```python
from build123d import *

# Parameters (mm, degrees)
SKETCH_1_W               = 10
SKETCH_1_H               = 10
SKETCH_1_W_2             = 8
SKETCH_1_H_2             = 8
EXTRUDE_1_DEPTH          = 121
SKETCH_2_R               = 1.5
CUT_EXTRUDE_1_DEPTH      = 11
SKETCH_3_R               = 1.5
CUT_EXTRUDE_2_DEPTH      = 51.396370289
CUT_EXTRUDE_2_DEPTH_BACK = 11.103629711


with BuildPart() as part:
    # 草图1 → 拉伸-薄壁1 (new body)
    with BuildSketch(Plane.XY):
        Rectangle(SKETCH_1_W, SKETCH_1_H)
        Rectangle(SKETCH_1_W_2, SKETCH_1_H_2, mode=Mode.SUBTRACT)
    extrude(amount=EXTRUDE_1_DEPTH)

    # 草图2 → 切除-拉伸1 (cut, through all)
    with BuildSketch(Plane(origin=(5, 0, 0), x_dir=(0, 0, -1), z_dir=(1, 0, 0))):
        with Locations((-103, 0)):
            Circle(SKETCH_2_R)
        with Locations((-35.5, 0)):
            Circle(SKETCH_2_R)
        with Locations((-25.5, 0)):
            Circle(SKETCH_2_R)
        with Locations((-93, 0)):
            Circle(SKETCH_2_R)
        Polygon((-112.339745962, 0), (-103.679491924, 5), (-121, 5), (-121, -5), (-109.452994616, -5), align=None)
        Polygon((-8.660254038, 0), (-17.320508076, -5), (0, -5), (0, 5), (-11.547005384, 5), align=None)
    extrude(amount=-CUT_EXTRUDE_1_DEPTH, mode=Mode.SUBTRACT)

    # 草图3 → 切除-拉伸2 (cut, two sides)
    with BuildSketch(Plane(origin=(0, 8.75, 5.051814855), x_dir=(1, 0, 0), z_dir=(0, 0.866025404, 0.5))) as cut_extrude_2_sk:
        with Locations((0, -12)):
            Circle(SKETCH_3_R)
    extrude(amount=CUT_EXTRUDE_2_DEPTH, mode=Mode.SUBTRACT)
    extrude(cut_extrude_2_sk.sketch, amount=-CUT_EXTRUDE_2_DEPTH_BACK, mode=Mode.SUBTRACT)


solid = part.part
```
Can you work these out from the model? Positions are in its coordinate system, mm. A direction names the side the tool comes from. Coordinates: 2 decimals unless noted, no trailing zeros. Loops run counter-clockwise (first coordinate to the right, second up) from the corner with the lowest first, then second, coordinate; pieces in that order, holes last. Notation, with made-up numbers: M 19,23 L 35,23 A18 cw 35,53 Z; hole C 54,-24.5 d5. An arc over 180 degrees is marked long. Put each result on its own line as item: value. Start each with the question number.
(1) We'd pull the mould along X, two halves only. Please class faces 1 (the face through (0, 4, 58)), 2 (the face through (4.51, 0.07, 27)), 3 (the face through (5, 0, 60)): +X half, -X half, draft (parallel to the pull), parting line (faces both ways), or undercut.
(2) Imagine slicing it at A-A on z = 25.5. List the corners of the cut face in (x, y) for me.
(3) Which directions (+Z, -Z, +X, -X, +Y, -Y) give clear straight access to the entire face, cutting with the end or side of a thin tool? Please do faces 4 (the face through (0, -4, 62)), 5 (the face through (-1.5, 4.55, 16.41)).
(4) I need wall thicknesses on probe 1 along X at (y, z) = (-2.5, 21); probe 2 along Y at (x, z) = (4.6, 93). Which ranges of each line are inside material? Lowest first, please.
(5) Will these pins go through, and if not, where does the flat tip stop? pin 1 Ø4 at (y, z) = (0, 35.5) entering from +X; pin 2 Ø1 at (x, y) = (-4, 1.5) entering from +Z.
(6) Imagine slicing it at C-C on z = 50. List the corners of the cut face in (x, y) for me, and give its area (3 significant figures).
(7) Imagine slicing it at B-B on y = 2.75. List the corners of the cut face in (x, z) for me, and give its area (3 significant figures).
Worked answers:
1. face 1: undercut
1. face 2: draft
1. face 3: +X half
2. outline: M -5,-5 L 5,-5 L 5,-1.5 L 4,-1.5 L 4,-4 L -4,-4 L -4,-1.5 L -5,-1.5 Z; M -5,1.5 L -4,1.5 L -4,4 L 4,4 L 4,1.5 L 5,1.5 L 5,5 L -5,5 Z
3. face 4: +Z, -Z
3. face 5: none
4. probe 1: x = -5 to -4, 4 to 5
4. probe 2: y = -5 to -1.5, 1.5 to 5
5. pin 1: stops at x = 5
5. pin 2: stops at z = 110.61
6. outline: M -5,-5 L 5,-5 L 5,5 L -5,5 Z; hole M -4,-4 L 4,-4 L 4,4 L -4,4 Z
6. area: 36.0 mm2
7. outline: M -5,10.25 L -4,10.25 L -4,107.58 L -5,107.58 Z; M 4,10.25 L 5,10.25 L 5,107.58 L 4,107.58 Z
7. area: 195 mm2
